```python
from build123d import *

# Parameters (mm, degrees)
SKETCH_W        = 115
SKETCH_H        = 62
PAD_DEPTH       = 30
SKETCH001_W     = 113
SKETCH001_H     = 58
POCKET_DEPTH    = 28
SKETCH002_R     = 3
PAD001_DEPTH    = 5
SKETCH003_R     = 1.375
SKETCH003_W     = 28
SKETCH003_H     = 20
POCKET001_DEPTH = 7
POCKET002_DEPTH = 2
SKETCH005_W     = 9.5
SKETCH005_H     = 4.4
SKETCH005_W_2   = 17
SKETCH005_H_2   = 8.3
SKETCH005_W_3   = 8.85
SKETCH005_H_3   = 8
POCKET003_DEPTH = 2
SKETCH006_W     = 62
SKETCH006_H     = 8
PAD002_DEPTH    = 2
POCKET004_DEPTH = 2
SKETCH010_R     = 3
PAD004_DEPTH    = 7
POCKET007_DEPTH = 2
SKETCH014_R     = 4
PAD005_DEPTH    = 30
SKETCH020_R     = 1.35
POCKET010_DEPTH = 7
SKETCH021_R     = 3
PAD006_DEPTH    = 7
SKETCH022_R     = 1.35
POCKET011_DEPTH = 7
SKETCH023_R     = 2
POCKET012_DEPTH = 30
SKETCH024_R     = 2
POCKET013_DEPTH = 30
SKETCH025_R     = 2
POCKET014_DEPTH = 30
SKETCH026_R     = 2
POCKET015_DEPTH = 30
POCKET016_DEPTH = 5
POCKET017_DEPTH = 5
POCKET018_DEPTH = 5
POCKET019_DEPTH = 5
FILLET_R        = 1


with BuildPart() as part:
    # Sketch → Pad (new body)
    with BuildSketch(Plane.XY):
        with Locations((27.5, 31)):
            Rectangle(SKETCH_W, SKETCH_H)
    extrude(amount=PAD_DEPTH)

    # Sketch001 (on Face6 of Pad) → Pocket (cut)
    with BuildSketch(Plane.XY.offset(30)):
        with Locations((28.5, 31)):
            Rectangle(SKETCH001_W, SKETCH001_H)
    extrude(amount=-POCKET_DEPTH, mode=Mode.SUBTRACT)

    # Sketch002 (on Face8 of Pocket) → Pad001 (join)
    with BuildSketch(Plane.XY.offset(2)):
        with Locations((3.5, 5.5)):
            Circle(SKETCH002_R)
        with Locations((61.5, 5.5)):
            Circle(SKETCH002_R)
        with Locations((3.5, 54.5)):
            Circle(SKETCH002_R)
        with Locations((61.5, 54.5)):
            Circle(SKETCH002_R)
        with Locations((-7, 45)):
            Circle(SKETCH002_R)
        with Locations((-24, 17)):
            Circle(SKETCH002_R)
    extrude(amount=PAD001_DEPTH)

    # Sketch003 (on Face21 of Pad001) → Pocket001 (cut)
    with BuildSketch(Plane.XY.offset(7)):
        with Locations((3.5, 54.5)):
            Circle(SKETCH003_R)
        with Locations((61.5, 54.5)):
            Circle(SKETCH003_R)
        with Locations((3.5, 5.5)):
            Circle(SKETCH003_R)
        with Locations((61.5, 5.5)):
            Circle(SKETCH003_R)
        with Locations((-7, 45)):
            Circle(SKETCH003_R)
        with Locations((-24, 17)):
            Circle(SKETCH003_R)
        with Locations((-6, 30)):
            Rectangle(SKETCH003_W, SKETCH003_H)
    extrude(amount=-POCKET001_DEPTH, mode=Mode.SUBTRACT)

    # Sketch004 (on Face4 of Pocket001) → Pocket002 (cut)
    with BuildSketch(Plane(origin=(0, 0, 0), x_dir=(1, 0, 0), z_dir=(0, 0, -1))):
        Polygon((4.75, -7.665064), (6, -5.5), (4.75, -3.334936), (2.25, -3.334936), (1, -5.5), (2.25, -7.665064), align=None)
        Polygon((62.75, -7.665064), (64, -5.5), (62.75, -3.334936), (60.25, -3.334936), (59, -5.5), (60.25, -7.665064), align=None)
        Polygon((62.75, -56.665064), (64, -54.5), (62.75, -52.334936), (60.25, -52.334936), (59, -54.5), (60.25, -56.665064), align=None)
        Polygon((4.75, -56.665064), (6, -54.5), (4.75, -52.334936), (2.25, -52.334936), (1, -54.5), (2.25, -56.665064), align=None)
        Polygon((-5.75, -47.165064), (-4.5, -45), (-5.75, -42.834936), (-8.25, -42.834936), (-9.5, -45), (-8.25, -47.165064), align=None)
        Polygon((-22.75, -19.165064), (-21.5, -17), (-22.75, -14.834936), (-25.25, -14.834936), (-26.5, -17), (-25.25, -19.165064), align=None)
    extrude(amount=-POCKET002_DEPTH, mode=Mode.SUBTRACT)

    # Sketch005 (on Face6 of Pocket002) → Pocket003 (cut)
    with BuildSketch(Plane.XZ):
        with Locations((10.6, 9.7)):
            Rectangle(SKETCH005_W, SKETCH005_H)
        with Locations((32, 11.65)):
            Rectangle(SKETCH005_W_2, SKETCH005_H_2)
        with Locations((53.5, 11.5)):
            Rectangle(SKETCH005_W_3, SKETCH005_H_3)
    extrude(amount=-POCKET003_DEPTH, mode=Mode.SUBTRACT)

    # Sketch006 (on Face3 of Pocket003) → Pad002 (join)
    with BuildSketch(Plane.YZ.offset(85)):
        with Locations((31, 4)):
            Rectangle(SKETCH006_W, SKETCH006_H)
    extrude(amount=PAD002_DEPTH)

    # Sketch007 (on Face2 of Pad002) → Pocket004 (cut)
    with BuildSketch(Plane(origin=(-30, 0, 0), x_dir=(0, -1, 0), z_dir=(-1, 0, 0))):
        with BuildLine():
            ThreePointArc((-50, 25), (-55, 20), (-50, 15))
            Line((-50, 15), (-40, 15))
            ThreePointArc((-40, 15), (-35, 20), (-40, 25))
            Line((-50, 25), (-40, 25))
        make_face()
    extrude(amount=-POCKET004_DEPTH, mode=Mode.SUBTRACT)

    # Sketch010 → Pad004 (join)
    with BuildSketch(Plane.XY.offset(7)):
        with Locations((-7, 45)):
            Circle(SKETCH010_R)
    extrude(amount=PAD004_DEPTH)

    # Sketch013 (on Face4 of Pocket001) → Pocket007 (cut)
    with BuildSketch(Plane(origin=(0, 0, 0), x_dir=(1, 0, 0), z_dir=(0, 0, -1))):
        Polygon((-22.75, -19.165064), (-21.5, -17), (-22.75, -14.834936), (-25.25, -14.834936), (-26.5, -17), (-25.25, -19.165064), align=None)
        Polygon((4.75, -7.665064), (6, -5.5), (4.75, -3.334936), (2.25, -3.334936), (1, -5.5), (2.25, -7.665064), align=None)
        Polygon((-5.75, -47.165064), (-4.5, -45), (-5.75, -42.834936), (-8.25, -42.834936), (-9.5, -45), (-8.25, -47.165064), align=None)
        Polygon((6, -54.5), (4.75, -52.334936), (2.25, -52.334936), (1, -54.5), (2.25, -56.665064), (4.75, -56.665064), align=None)
        Polygon((64, -54.5), (62.75, -52.334936), (60.25, -52.334936), (59, -54.5), (60.25, -56.665064), (62.75, -56.665064), align=None)
        Polygon((64, -5.5), (62.75, -3.334936), (60.25, -3.334936), (59, -5.5), (60.25, -7.665064), (62.75, -7.665064), align=None)
    extrude(amount=-POCKET007_DEPTH, mode=Mode.SUBTRACT)

    # Sketch014 (on Face5 of Pocket007) → Pad005 (join)
    with BuildSketch(Plane(origin=(0, 0, 0), x_dir=(1, 0, 0), z_dir=(0, 0, -1))):
        with Locations((-24, 2)):
            Circle(SKETCH014_R)
        with Locations((81, 2)):
            Circle(SKETCH014_R)
        with Locations((-24, -64)):
            Circle(SKETCH014_R)
        with Locations((81, -64)):
            Circle(SKETCH014_R)
    extrude(amount=-PAD005_DEPTH)

    # Sketch020 → Pocket010 (cut)
    with BuildSketch(Plane.XY.offset(14)):
        with Locations((-7, 45)):
            Circle(SKETCH020_R)
    extrude(amount=-POCKET010_DEPTH, mode=Mode.SUBTRACT)

    # Sketch021 (on Face130 of Pocket010) → Pad006 (join)
    with BuildSketch(Plane.XY.offset(7)):
        with Locations((-24, 17)):
            Circle(SKETCH021_R)
    extrude(amount=PAD006_DEPTH)

    # Sketch022 (on Face136 of Pad006) → Pocket011 (cut)
    with BuildSketch(Plane.XY.offset(14)):
        with Locations((-24, 17)):
            Circle(SKETCH022_R)
    extrude(amount=-POCKET011_DEPTH, mode=Mode.SUBTRACT)

    # Sketch023 (on Face57 of Pocket011) → Pocket012 (cut)
    with BuildSketch(Plane.XY.offset(30)):
        with Locations((-24, 64)):
            Circle(SKETCH023_R)
    extrude(amount=-POCKET012_DEPTH, mode=Mode.SUBTRACT)

    # Sketch024 (on Face115 of Pocket012) → Pocket013 (cut)
    with BuildSketch(Plane.XY.offset(30)):
        with Locations((81, 64)):
            Circle(SKETCH024_R)
    extrude(amount=-POCKET013_DEPTH, mode=Mode.SUBTRACT)

    # Sketch025 (on Face110 of Pocket013) → Pocket014 (cut)
    with BuildSketch(Plane.XY.offset(30)):
        with Locations((81, -2)):
            Circle(SKETCH025_R)
    extrude(amount=-POCKET014_DEPTH, mode=Mode.SUBTRACT)

    # Sketch026 (on Face106 of Pocket014) → Pocket015 (cut)
    with BuildSketch(Plane.XY.offset(30)):
        with Locations((-24, -2)):
            Circle(SKETCH026_R)
    extrude(amount=-POCKET015_DEPTH, mode=Mode.SUBTRACT)

    # Sketch027 (on Face69 of Pocket015) → Pocket016 (cut)
    with BuildSketch(Plane(origin=(0, 0, 0), x_dir=(1, 0, 0), z_dir=(0, 0, -1))):
        Polygon((-21.125, 2), (-22.5625, 4.489823), (-25.4375, 4.489823), (-26.875, 2), (-25.4375, -0.489823), (-22.5625, -0.489823), align=None)
    extrude(amount=-POCKET016_DEPTH, mode=Mode.SUBTRACT)

    # Sketch028 (on Face88 of Pocket016) → Pocket017 (cut)
    with BuildSketch(Plane(origin=(0, 0, 0), x_dir=(1, 0, 0), z_dir=(0, 0, -1))):
        Polygon((82.4375, 4.489823), (79.5625, 4.489823), (78.125, 2), (79.5625, -0.489823), (82.4375, -0.489823), (83.875, 2), align=None)
    extrude(amount=-POCKET017_DEPTH, mode=Mode.SUBTRACT)

    # Sketch029 (on Face101 of Pocket017) → Pocket018 (cut)
    with BuildSketch(Plane(origin=(0, 0, 0), x_dir=(1, 0, 0), z_dir=(0, 0, -1))):
        Polygon((82.4375, -66.489823), (83.875, -64), (82.4375, -61.510177), (79.5625, -61.510177), (78.125, -64), (79.5625, -66.489823), align=None)
    extrude(amount=-POCKET018_DEPTH, mode=Mode.SUBTRACT)

    # Sketch030 (on Face58 of Pocket018) → Pocket019 (cut)
    with BuildSketch(Plane(origin=(0, 0, 0), x_dir=(1, 0, 0), z_dir=(0, 0, -1))):
        Polygon((-22.5625, -66.489823), (-21.125, -64), (-22.5625, -61.510177), (-25.4375, -61.510177), (-26.875, -64), (-25.4375, -66.489823), align=None)
    extrude(amount=-POCKET019_DEPTH, mode=Mode.SUBTRACT)

    # Fillet
    fillet_edges = [part.edges().sort_by_distance(p)[0] for p in [
        (32, 0, 7.5),
        (32, 0, 15.8),
        (23.5, 0, 11.65),
        (40.5, 0, 11.65),
        (10.6, 0, 11.9),
        (10.6, 0, 7.5),
        (15.35, 0, 9.7),
        (5.85, 0, 9.7),
        (49.075, 0, 11.5),
        (53.5, 0, 7.5),
        (57.925, 0, 11.5),
        (53.5, 0, 15.5),
        (-30, 45, 15),
        (-30, 45, 25),
        (-30, 62, 15),
        (-30, 0, 15),
        (-30, 31, 0),
        (87, 31, 0),
        (-30, 35, 20),
        (-30, 55, 20),
    ]]
    fillet(fillet_edges, radius=FILLET_R)


solid = part.part
```
Input: part model. Units: mm. Frame: model coordinates. A direction names the side the tool comes from. Round coordinates to 2 decimals unless told otherwise and drop trailing zeros. Loops run counter-clockwise (first coordinate to the right, second up) from the corner with the lowest first, then second, coordinate; pieces in that order, holes last. Notation, with made-up numbers: M -10,69 L 47,69 A16 cw 47,98 Z; hole C 14.25,-8.5 d11. An arc over 180 degrees is marked long. Answer in a Markdown table with one row per item. Add a question column.
1. Mould query, pull axis Y, two halves, no side actions, for faces 4 (the face through (-28.5, 55, 20.1)), 5 (the face through (-30, 31, 15)). Classes: released by +Y, released by -Y, zero draft, split by the parting line, or undercut.
2. Section B-B (x = 26.5). Output: boundary loops of the cut face in (y, z).
3. Contact query for flat-ended pins moving along their axis: pin 1 (6 mm diameter, centred on x = -4.5, z = 11, fed in from -Y); pin 2 (1.4 mm diameter, centred on x = -23.5, y = 17, fed in from -Z); pin 3 (4 mm diameter, centred on y = 55.5, z = 11.5, fed in from +X); pin 4 (1.6 mm diameter, centred on x = 86.5, y = 33, fed in from +Z). Output: stop coordinate, or through.
4. Section D-D (y = 12). Output: boundary loops of the cut face in (x, z), and give its area (3 significant figures).
5. Section A-A (y = 32.5). Output: boundary loops of the cut face in (x, z).
6. Set-up query: faces 1 (the face through (28, 2, 16)), 2 (the face through (-26, -2, 18)), 3 (the face through (78.834, -0.773, 2.465)). Return all of +Z, -Z, +X, -X, +Y, -Y with unobstructed straight access to the full face (end or side cutting, diameter ignored); none if empty.
7. Ray query, probe 1 along Y at (x, z) = (3.5, 3.95) (3 decimals); probe 2 along Y at (x, z) = (61.5, 12.75); probe 3 along Y at (x, z) = (-7, 9.75). Return the intervals inside material, ascending.
8. Section C-C (x = -7). Output: boundary loops of the cut face in (y, z) (3 decimals).
Values follow:
| question | item | result |
|---|---|---|
| 1 | face 4 | undercut |
| 1 | face 5 | zero draft |
| 2 | outline | M 0,0 L 62,0 L 62,30 L 60,30 L 60,2 L 2,2 L 2,7.5 L 1,7.5 A1 ccw 0,6.5 Z; M 0,16.8 A1 ccw 1,15.8 L 2,15.8 L 2,30 L 0,30 Z |
| 3 | pin 1 | y = 0 |
| 3 | pin 2 | through |
| 3 | pin 3 | x = -28 |
| 3 | pin 4 | z = 8 |
| 4 | outline | M -30,1 A1 ccw -29,0 L 86,0 A1 ccw 87,1 L 87,8 L 85,8 L 85,2 L -28,2 L -28,30 L -30,30 Z |
| 4 | area | 302 mm^2 |
| 5 | outline | M -30,1 A1 ccw -29,0 L -20,0 L -20,2 L -28,2 L -28,30 L -30,30 Z; M 8,0 L 86,0 A1 ccw 87,1 L 87,8 L 85,8 L 85,2 L 8,2 Z |
| 6 | face 1 | +Z |
| 6 | face 2 | +Z, -Z |
| 6 | face 3 | -Z |
| 7 | probe 1 | 0 to 2, 2.5 to 4.125, 6.875 to 8.5, 51.5 to 53.125, 55.875 to 57.5, 60 to 62 |
| 7 | probe 2 | 0 to 2, 60 to 62 |
| 7 | probe 3 | 0 to 2, 42 to 43.65, 46.35 to 48, 60 to 62 |
| 8 | outline | M 0,0 L 20,0 L 20,2 L 2,2 L 2,30 L 0,30 Z; M 40,0 L 42.835,0 L 42.835,2 L 43.625,2 L 43.625,7 L 43.65,7 L 43.65,14 L 42,14 L 42,2 L 40,2 Z; M 46.35,7 L 46.375,7 L 46.375,2 L 47.165,2 L 47.165,0 L 62,0 L 62,30 L 60,30 L 60,2 L 48,2 L 48,14 L 46.35,14 Z |
